Geometry: final body of the model. Coordinates: model frame, mm. Face numbers are marked on the shaded views. A direction names the side the tool comes from. Give positions to 0.01 mm unless a question says otherwise; leave off trailing zeros. Loops run counter-clockwise (first coordinate to the right, second up) from the corner with the lowest first, then second, coordinate; pieces in that order, holes last. Notation, with made-up numbers: M 7,39 L 61,39 A29 ccw 61,73 Z; hole C 12,61 d1. An arc over 180 degrees is marked long. Put each result on its own line as item: value.
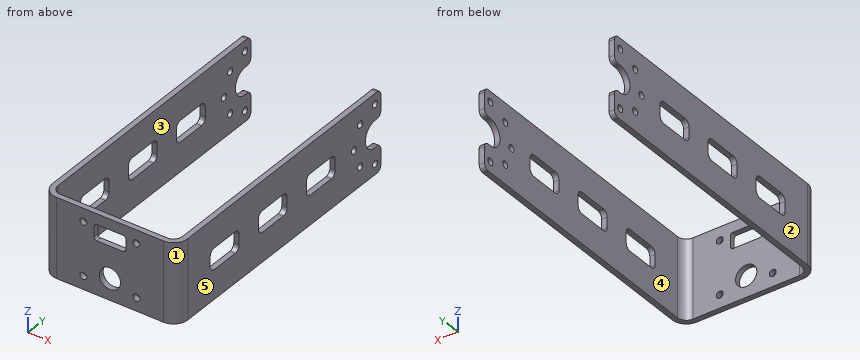
```python
from build123d import *

# Parameters (mm, degrees)
BASE_FLANGE1_DEPTH      = 15
CUT_EXTRUDE1_DEPTH      = 10
CUT_EXTRUDE2_DEPTH      = 108.837563029
CUT_EXTRUDE2_DEPTH_BACK = 108.837563029
SKETCH6_R               = 1.3
SKETCH8_R               = 4
SKETCH8_W               = 12
SKETCH8_H               = 6
CUT_EXTRUDE4_DEPTH      = 10
CUT_EXTRUDE5_DEPTH      = 108.837563029
CUT_EXTRUDE5_DEPTH_BACK = 108.837563029
FILLET1_R               = 2
FILLET2_R               = 1


# Sheet-metal steps are written as plain solids
with BuildPart() as part:
    # Sketch1 → Base-Flange1 (new, symmetric)
    with BuildSketch(Plane.XY):
        with BuildLine():
            Line((-23.5, 103.7), (-23.5, 3.33))
            ThreePointArc((-23.5, 3.33), (-22.524665581, 0.975334419), (-20.17, 0))
            Line((-20.17, 0), (20.17, 0))
            ThreePointArc((20.17, 0), (22.524665581, 0.975334419), (23.5, 3.33))
            Line((23.5, 3.33), (23.5, 103.7))
            Line((23.5, 103.7), (25.5, 103.7))
            Line((25.5, 103.7), (25.5, 3.33))
            ThreePointArc((25.5, 3.33), (23.938879144, -0.438879144), (20.17, -2))
            Line((20.17, -2), (-20.17, -2))
            ThreePointArc((-20.17, -2), (-23.938879144, -0.438879144), (-25.5, 3.33))
            Line((-25.5, 3.33), (-25.5, 103.7))
            Line((-25.5, 103.7), (-23.5, 103.7))
        make_face()
    extrude(amount=BASE_FLANGE1_DEPTH, both=True)

    # Sketch5 → Cut-Extrude1 (cut)
    with BuildSketch(Plane.XZ.offset(2)):
        with BuildLine():
            Line((-10, 8.7), (-10, 10))
            Line((-10, 10), (-8.7, 10))
            ThreePointArc((-8.7, 10), (-10.919238816, 10.919238816), (-10, 8.7))
        make_face()
        with BuildLine():
            Line((-8.7, 10), (-10, 10))
            Line((-10, 10), (-10, 8.7))
            ThreePointArc((-10, 8.7), (-9.080761184, 9.080761184), (-8.7, 10))
        make_face()
        with BuildLine():
            ThreePointArc((11.3, 10), (10, 11.3), (8.7, 10))
            Line((8.7, 10), (10, 10))
            Line((10, 10), (10, 8.7))
            ThreePointArc((10, 8.7), (10.919238816, 9.080761184), (11.3, 10))
        make_face()
        with BuildLine():
            Line((10, 10), (8.7, 10))
            ThreePointArc((8.7, 10), (9.080761184, 9.080761184), (10, 8.7))
            Line((10, 8.7), (10, 10))
        make_face()
        with BuildLine():
            ThreePointArc((11.3, -10), (10.919238816, -9.080761184), (10, -8.7))
            Line((10, -8.7), (10, -10))
            Line((10, -10), (8.7, -10))
            ThreePointArc((8.7, -10), (10, -11.3), (11.3, -10))
        make_face()
        with BuildLine():
            Line((10, -10), (10, -8.7))
            ThreePointArc((10, -8.7), (9.080761184, -9.080761184), (8.7, -10))
            Line((8.7, -10), (10, -10))
        make_face()
        with BuildLine():
            ThreePointArc((-8.7, -10), (-9.080761184, -9.080761184), (-10, -8.7))
            Line((-10, -8.7), (-10, -10))
            Line((-10, -10), (-8.7, -10))
        make_face()
        with BuildLine():
            Line((-10, -10), (-10, -8.7))
            ThreePointArc((-10, -8.7), (-10.919238816, -10.919238816), (-8.7, -10))
            Line((-8.7, -10), (-10, -10))
        make_face()
    extrude(amount=-CUT_EXTRUDE1_DEPTH, mode=Mode.SUBTRACT)

    # Sketch6 → Cut-Extrude2 (cut, two sides: drawn at the far end of the back side and taken through both)
    with BuildSketch(Plane(origin=(0, 0, 0), x_dir=(0, 0, -1), z_dir=(1, 0, 0)).offset(-CUT_EXTRUDE2_DEPTH_BACK)):
        with BuildLine():
            ThreePointArc((-4.062326919, 103.7), (-4.796730707, 102.279200598), (-5.05, 100.7))
            ThreePointArc((-5.05, 100.7), (0, 95.65), (5.05, 100.7))
            ThreePointArc((5.05, 100.7), (4.796730707, 102.279200598), (4.062326919, 103.7))
            Line((4.062326919, 103.7), (-4.062326919, 103.7))
        make_face()
        with BuildLine():
            ThreePointArc((4.062326919, 103.7), (0, 105.75), (-4.062326919, 103.7))
            Line((-4.062326919, 103.7), (4.062326919, 103.7))
        make_face()
        with BuildLine():
            Line((-5.05, 103.7), (-5.05, 100.7))
            ThreePointArc((-5.05, 100.7), (-4.796730707, 102.279200598), (-4.062326919, 103.7))
            Line((-4.062326919, 103.7), (-5.05, 103.7))
        make_face()
        with BuildLine():
            ThreePointArc((4.062326919, 103.7), (4.796730707, 102.279200598), (5.05, 100.7))
            Line((5.05, 100.7), (5.05, 103.7))
            Line((5.05, 103.7), (4.062326919, 103.7))
        make_face()
        with Locations(Location((11, 100.7, 0), (0, 0, 90))):
            Circle(SKETCH6_R)
        with Locations(Location((0, 89.7, 0), (0, 0, 90))):
            Circle(SKETCH6_R)
        with Locations(Location((-7.778174593, 92.921825407, 0), (0, 0, 90))):
            Circle(SKETCH6_R)
        with Locations(Location((7.778174593, 92.921825407, 0), (0, 0, 90))):
            Circle(SKETCH6_R)
        with Locations(Location((-11, 100.7, 0), (0, 0, 90))):
            Circle(SKETCH6_R)
    extrude(amount=CUT_EXTRUDE2_DEPTH + CUT_EXTRUDE2_DEPTH_BACK, mode=Mode.SUBTRACT)

    # Sketch8 → Cut-Extrude4 (cut)
    with BuildSketch(Plane(origin=(0, 0, 0), x_dir=(1, 0, 0), z_dir=(0, 1, 0))):
        with Locations(Location((0, 7, 0), (0, 0, 270))):
            Circle(SKETCH8_R)
        with Locations((0, -8)):
            Rectangle(SKETCH8_W, SKETCH8_H)
    extrude(amount=-CUT_EXTRUDE4_DEPTH, mode=Mode.SUBTRACT)

    # Sketch9 → Cut-Extrude5 (cut, two sides: drawn at the far end of the back side and taken through both)
    with BuildSketch(Plane(origin=(0, 0, 0), x_dir=(0, 0, -1), z_dir=(1, 0, 0)).offset(-CUT_EXTRUDE5_DEPTH_BACK)):
        with BuildLine():
            Line((-2, 40), (2, 40))
            ThreePointArc((2, 40), (3.414213562, 40.585786438), (4, 42))
            Line((4, 42), (4, 53))
            ThreePointArc((4, 53), (3.414213562, 54.414213562), (2, 55))
            Line((2, 55), (-2, 55))
            ThreePointArc((-2, 55), (-3.414213562, 54.414213562), (-4, 53))
            Line((-4, 53), (-4, 42))
            ThreePointArc((-4, 42), (-3.414213562, 40.585786438), (-2, 40))
        make_face()
        with BuildLine():
            Line((-2, 15), (2, 15))
            ThreePointArc((2, 15), (3.414213562, 15.585786438), (4, 17))
            Line((4, 17), (4, 28))
            ThreePointArc((4, 28), (3.414213562, 29.414213562), (2, 30))
            Line((2, 30), (-2, 30))
            ThreePointArc((-2, 30), (-3.414213562, 29.414213562), (-4, 28))
            Line((-4, 28), (-4, 17))
            ThreePointArc((-4, 17), (-3.414213562, 15.585786438), (-2, 15))
        make_face()
        with BuildLine():
            Line((-2, 65), (2, 65))
            ThreePointArc((2, 65), (3.414213562, 65.585786438), (4, 67))
            Line((4, 67), (4, 78))
            ThreePointArc((4, 78), (3.414213562, 79.414213562), (2, 80))
            Line((2, 80), (-2, 80))
            ThreePointArc((-2, 80), (-3.414213562, 79.414213562), (-4, 78))
            Line((-4, 78), (-4, 67))
            ThreePointArc((-4, 67), (-3.414213562, 65.585786438), (-2, 65))
        make_face()
    extrude(amount=CUT_EXTRUDE5_DEPTH + CUT_EXTRUDE5_DEPTH_BACK, mode=Mode.SUBTRACT)

    # Fillet1
    fillet1_edges = [part.edges().sort_by_distance(p)[0] for p in [
        (-24.5, 103.7, -15),
        (24.5, 103.7, -15),
        (-24.5, 103.7, 15),
        (24.5, 103.7, 15),
        (24.5, 103.7, -5.05),
        (24.5, 103.7, 5.05),
        (-24.5, 103.7, -5.05),
        (-24.5, 103.7, 5.05),
    ]]
    fillet(fillet1_edges, radius=FILLET1_R)

    # Fillet2
    fillet2_edges = [part.edges().sort_by_distance(p)[0] for p in [
        (-6, -1, 11),
        (-6, -1, 5),
        (6, -1, 5),
        (6, -1, 11),
    ]]
    fillet(fillet2_edges, radius=FILLET2_R)


solid = part.part
```
Item 1: Mould query, pull axis X, two halves, no side actions, for the marked faces 1, 2 and 3. Classes: pulls with the +X half, pulls with the -X half, needs draft (parallel to the pull), parting line crosses it, or undercut.
Output values:
face 1: pulls with the +X half
face 2: pulls with the -X half
face 3: undercut
Item 2: Section C-C on y = 89.7. Output: boundary loops of the cut face in (x, z), then the cut area to 3 significant figures.
Output values:
outline: M -25.5,-15 L -23.5,-15 L -23.5,-1.3 L -25.5,-1.3 Z; M -25.5,1.3 L -23.5,1.3 L -23.5,15 L -25.5,15 Z; M 23.5,-15 L 25.5,-15 L 25.5,-1.3 L 23.5,-1.3 Z; M 23.5,1.3 L 25.5,1.3 L 25.5,15 L 23.5,15 Z
area: 110 mm²
Item 3: Set-up query: the marked faces 4 and 5. Return all of +Z, -Z, +X, -X, +Y, -Y with unobstructed straight access to the full face (end or side cutting, diameter ignored); none if empty.
Output values:
face 4: +Z, -Z, +Y
face 5: +Z, -Z, +X, +Y, -Y
Item 4: Line query: probe 1 along Z at (x, y) = (-24.65, 100.7); probe 2 along X at (y, z) = (58, 10); probe 3 along X at (y, z) = (-0.5, -10). Output: solid intervals per line, ascending. Write a range as [from, to].
Output values:
probe 1: [-15, -12.3], [-9.7, -5.05], [5.05, 9.7], [12.3, 15]
probe 2: [-25.5, -23.5], [23.5, 25.5]
probe 3: [-23.88, -11.3], [-8.7, -2.65], [2.65, 8.7], [11.3, 23.88]
Item 5: Section A-A on y = 5.5. Output: boundary loops of the cut face in (x, z).
Output values:
outline: M -25.5,-15 L -23.5,-15 L -23.5,15 L -25.5,15 Z; M 23.5,-15 L 25.5,-15 L 25.5,15 L 23.5,15 Z
Item 6: Section D-D on y = 69. Output: boundary loops of the cut face in (x, z), then the cut area to 3 significant figures.
Output values:
outline: M -25.5,-15 L -23.5,-15 L -23.5,-4 L -25.5,-4 Z; M -25.5,4 L -23.5,4 L -23.5,15 L -25.5,15 Z; M 23.5,-15 L 25.5,-15 L 25.5,-4 L 23.5,-4 Z; M 23.5,4 L 25.5,4 L 25.5,15 L 23.5,15 Z
area: 88.0 mm²
Item 7: Section B-B on x = 0. Output: boundary loops of the cut face in (y, z), then the cut area to 3 significant figures.
Output values:
outline: M -2,-15 L 0,-15 L 0,-11 L -2,-11 Z; M -2,-3 L 0,-3 L 0,5 L -2,5 Z; M -2,11 L 0,11 L 0,15 L -2,15 Z
area: 32.0 mm²
Item 8: Pin query (flat end, axial travel): pin 1 Ø2 at (x, z) = (17, -7) entering from +Y; pin 2 Ø1.6 at (y, z) = (-1, 9) entering from +X; pin 3 Ø0.6 at (x, z) = (25, -0.5) entering from +Y. Return the tip coordinate at first contact, or that it passes through.
Output values:
pin 1: y = 0
pin 2: x = 24.16
pin 3: y = 95.71
